Geometry: final body of the model. Coordinates: model frame, mm. Face numbers are marked on the shaded views. Give positions to 0.01 mm unless a question says otherwise; leave off trailing zeros. Loops run counter-clockwise (first coordinate to the right, second up) from the corner with the lowest first, then second, coordinate; pieces in that order, holes last.
from build123d import *

# Parameters (mm, degrees)
F0_W         = 28
F0_H         = 88.9
F0_R         = 11.5
F1_DEPTH     = 11
F2_T1_DEPTH  = 78.74
F2_T3_DEPTH  = 17.84
F2_T5_DEPTH  = 0.84
F2_S9_W      = 5.08
F2_S9_H      = 5.08
F2_T10_DEPTH = 5.08
F2_S15_W     = 5.08
F2_S15_H     = 5.08
F2_T16_DEPTH = 5.08
F2_S21_W     = 5.08
F2_S21_H     = 5.08
F2_T22_DEPTH = 5.08
F2_S27_W     = 5.08
F2_S27_H     = 5.08
F2_T28_DEPTH = 5.08
F2_S33_W     = 5.08
F2_S33_H     = 5.08
F2_T34_DEPTH = 5.08
F2_S39_W     = 5.08
F2_S39_H     = 5.08
F2_T40_DEPTH = 5.08
F2_S45_W     = 5.08
F2_S45_H     = 5.08
F2_T46_DEPTH = 5.08
F2_S51_W     = 5.08
F2_S51_H     = 5.08
F2_T52_DEPTH = 5.08


# Not quite as in the source:
# - a fillet or chamfer that OpenCascade refuses, or shapes differently, is made with other operations: its cross-section is extruded or revolved along the edge and cut away or added


with BuildPart() as f1:
    # F0 (on Top) → F1 (new body)
    with BuildSketch(Plane.XY):
        with Locations((-14, 0)):
            Rectangle(F0_W, F0_H)
        with Locations((-13.97, -26.67)):
            Circle(F0_R, mode=Mode.SUBTRACT)
        with Locations((-13.97, 0)):
            Circle(F0_R, mode=Mode.SUBTRACT)
        with Locations((-13.97, 26.67)):
            Circle(F0_R, mode=Mode.SUBTRACT)
    extrude(amount=F1_DEPTH)

    # F2: fillet of radius 5.08 on 12 edges, made by hand

    # F2_s2 → F2_t1 (cut)
    with BuildSketch(Plane.XZ.offset(-39.37)):
        with BuildLine():
            ThreePointArc((0, 5.92), (-1.4878975516, 9.5121024484), (-5.08, 11))
            Line((-5.08, 11), (0, 11))
            Line((0, 11), (0, 5.92))
        make_face()
        with BuildLine():
            ThreePointArc((0, 5.08), (-1.4878975516, 1.4878975516), (-5.08, 0))
            Line((-5.08, 0), (0, 0))
            Line((0, 0), (0, 5.08))
        make_face()
        with BuildLine():
            ThreePointArc((-28, 5.92), (-26.5121024484, 9.5121024484), (-22.92, 11))
            Line((-22.92, 11), (-28, 11))
            Line((-28, 11), (-28, 5.92))
        make_face()
        with BuildLine():
            ThreePointArc((-28, 5.08), (-26.5121024484, 1.4878975516), (-22.92, 0))
            Line((-22.92, 0), (-28, 0))
            Line((-28, 0), (-28, 5.08))
        make_face()
    extrude(amount=F2_T1_DEPTH, mode=Mode.SUBTRACT)

    # F2_s4 → F2_t3 (cut)
    with BuildSketch(Plane.YZ.offset(-22.92)):
        with BuildLine():
            ThreePointArc((-44.45, 5.92), (-42.9621024484, 9.5121024484), (-39.37, 11))
            Line((-39.37, 11), (-44.45, 11))
            Line((-44.45, 11), (-44.45, 5.92))
        make_face()
        with BuildLine():
            ThreePointArc((-44.45, 5.08), (-42.9621024484, 1.4878975516), (-39.37, 0))
            Line((-39.37, 0), (-44.45, 0))
            Line((-44.45, 0), (-44.45, 5.08))
        make_face()
        with BuildLine():
            ThreePointArc((44.45, 5.92), (42.9621024484, 9.5121024484), (39.37, 11))
            Line((39.37, 11), (44.45, 11))
            Line((44.45, 11), (44.45, 5.92))
        make_face()
        with BuildLine():
            ThreePointArc((44.45, 5.08), (42.9621024484, 1.4878975516), (39.37, 0))
            Line((39.37, 0), (44.45, 0))
            Line((44.45, 0), (44.45, 5.08))
        make_face()
    extrude(amount=F2_T3_DEPTH, mode=Mode.SUBTRACT)

    # F2_s6 → F2_t5 (cut)
    with BuildSketch(Plane.XY.offset(5.08)):
        with BuildLine():
            ThreePointArc((0, -39.37), (-1.4878975516, -42.9621024484), (-5.08, -44.45))
            Line((-5.08, -44.45), (0, -44.45))
            Line((0, -44.45), (0, -39.37))
        make_face()
        with BuildLine():
            ThreePointArc((-28, -39.37), (-26.5121024484, -42.9621024484), (-22.92, -44.45))
            Line((-22.92, -44.45), (-28, -44.45))
            Line((-28, -44.45), (-28, -39.37))
        make_face()
        with BuildLine():
            ThreePointArc((-22.92, 44.45), (-26.5121024484, 42.9621024484), (-28, 39.37))
            Line((-28, 39.37), (-28, 44.45))
            Line((-28, 44.45), (-22.92, 44.45))
        make_face()
        with BuildLine():
            ThreePointArc((0, 39.37), (-1.4878975516, 42.9621024484), (-5.08, 44.45))
            Line((-5.08, 44.45), (0, 44.45))
            Line((0, 44.45), (0, 39.37))
        make_face()
    extrude(amount=F2_T5_DEPTH, mode=Mode.SUBTRACT)


with BuildPart() as f2_tool8:
    # F2_s9 → F2_t10 (new body)
    with BuildSketch(Plane.YZ.offset(-5.08)):
        with Locations((-41.91, 8.46)):
            Rectangle(F2_S9_W, F2_S9_H)
    extrude(amount=F2_T10_DEPTH)

    # F2_s11 → F2_t12 (revolve, cut)
    with BuildSketch(Plane(origin=(-5.08, -39.37, 5.92), x_dir=(0, 0.7071067812, -0.7071067812), z_dir=(0, -0.7071067812, -0.7071067812))):
        with BuildLine():
            ThreePointArc((0, -5.08), (5.08, 0), (0, 5.08))
            Line((0, 5.08), (0, -5.08))
        make_face()
    revolve(axis=Axis((-5.08, -39.37, 5.92), (1, 0, 0)), mode=Mode.SUBTRACT)


with BuildPart() as f1_1:
    add(f1.part)

    # F2_t7: cut F2_tool8
    add(f2_tool8.part, mode=Mode.SUBTRACT)


with BuildPart() as f2_tool14:
    # F2_s15 → F2_t16 (new body)
    with BuildSketch(Plane.YZ.offset(-5.08)):
        with Locations((41.91, 8.46)):
            Rectangle(F2_S15_W, F2_S15_H)
    extrude(amount=F2_T16_DEPTH)

    # F2_s17 → F2_t18 (revolve, cut)
    with BuildSketch(Plane(origin=(-5.08, 39.37, 5.92), x_dir=(0, -0.7071067812, -0.7071067812), z_dir=(0, -0.7071067812, 0.7071067812))):
        with BuildLine():
            ThreePointArc((0, -5.08), (5.08, 0), (0, 5.08))
            Line((0, 5.08), (0, -5.08))
        make_face()
    revolve(axis=Axis((-5.08, 39.37, 5.92), (1, 0, 0)), mode=Mode.SUBTRACT)


with BuildPart() as f1_2:
    add(f1_1.part)

    # F2_t13: cut F2_tool14
    add(f2_tool14.part, mode=Mode.SUBTRACT)


with BuildPart() as f2_tool20:
    # F2_s21 → F2_t22 (new body)
    with BuildSketch(Plane.XY.offset(5.92)):
        with Locations((-25.46, -41.91)):
            Rectangle(F2_S21_W, F2_S21_H)
    extrude(amount=F2_T22_DEPTH)

    # F2_s23 → F2_t24 (revolve, cut)
    with BuildSketch(Plane(origin=(-22.92, -39.37, 5.92), x_dir=(0.7071067812, 0.7071067812, 0), z_dir=(0.7071067812, -0.7071067812, 0))):
        with BuildLine():
            ThreePointArc((0, -5.08), (5.08, 0), (0, 5.08))
            Line((0, 5.08), (0, -5.08))
        make_face()
    revolve(axis=Axis((-22.92, -39.37, 5.92), (0, 0, 1)), mode=Mode.SUBTRACT)


with BuildPart() as f1_3:
    add(f1_2.part)

    # F2_t19: cut F2_tool20
    add(f2_tool20.part, mode=Mode.SUBTRACT)


with BuildPart() as f2_tool26:
    # F2_s27 → F2_t28 (new body)
    with BuildSketch(Plane.YZ.offset(-22.92)):
        with Locations((-41.91, 2.54)):
            Rectangle(F2_S27_W, F2_S27_H)
    extrude(amount=-F2_T28_DEPTH)

    # F2_s29 → F2_t30 (revolve, cut)
    with BuildSketch(Plane(origin=(-22.92, -39.37, 5.08), x_dir=(0, 0.7071067812, 0.7071067812), z_dir=(0, -0.7071067812, 0.7071067812))):
        with BuildLine():
            ThreePointArc((0, -5.08), (5.08, 0), (0, 5.08))
            Line((0, 5.08), (0, -5.08))
        make_face()
    revolve(axis=Axis((-22.92, -39.37, 5.08), (-1, 0, 0)), mode=Mode.SUBTRACT)


with BuildPart() as f1_4:
    add(f1_3.part)

    # F2_t25: cut F2_tool26
    add(f2_tool26.part, mode=Mode.SUBTRACT)


with BuildPart() as f2_tool32:
    # F2_s33 → F2_t34 (new body)
    with BuildSketch(Plane.YZ.offset(-5.08)):
        with Locations((-41.91, 2.54)):
            Rectangle(F2_S33_W, F2_S33_H)
    extrude(amount=F2_T34_DEPTH)

    # F2_s35 → F2_t36 (revolve, cut)
    with BuildSketch(Plane(origin=(-5.08, -39.37, 5.08), x_dir=(0, 0.7071067812, 0.7071067812), z_dir=(0, 0.7071067812, -0.7071067812))):
        with BuildLine():
            ThreePointArc((0, -5.08), (5.08, 0), (0, 5.08))
            Line((0, 5.08), (0, -5.08))
        make_face()
    revolve(axis=Axis((-5.08, -39.37, 5.08), (1, 0, 0)), mode=Mode.SUBTRACT)


with BuildPart() as f1_5:
    add(f1_4.part)

    # F2_t31: cut F2_tool32
    add(f2_tool32.part, mode=Mode.SUBTRACT)


with BuildPart() as f2_tool38:
    # F2_s39 → F2_t40 (new body)
    with BuildSketch(Plane.YZ.offset(-5.08)):
        with Locations((41.91, 2.54)):
            Rectangle(F2_S39_W, F2_S39_H)
    extrude(amount=F2_T40_DEPTH)

    # F2_s41 → F2_t42 (revolve, cut)
    with BuildSketch(Plane(origin=(-5.08, 39.37, 5.08), x_dir=(0, -0.7071067812, 0.7071067812), z_dir=(0, 0.7071067812, 0.7071067812))):
        with BuildLine():
            ThreePointArc((0, -5.08), (5.08, 0), (0, 5.08))
            Line((0, 5.08), (0, -5.08))
        make_face()
    revolve(axis=Axis((-5.08, 39.37, 5.08), (1, 0, 0)), mode=Mode.SUBTRACT)


with BuildPart() as f1_6:
    add(f1_5.part)

    # F2_t37: cut F2_tool38
    add(f2_tool38.part, mode=Mode.SUBTRACT)


with BuildPart() as f2_tool44:
    # F2_s45 → F2_t46 (new body)
    with BuildSketch(Plane.XY.offset(5.92)):
        with Locations((-25.46, 41.91)):
            Rectangle(F2_S45_W, F2_S45_H)
    extrude(amount=F2_T46_DEPTH)

    # F2_s47 → F2_t48 (revolve, cut)
    with BuildSketch(Plane(origin=(-22.92, 39.37, 5.92), x_dir=(0.7071067812, -0.7071067812, 0), z_dir=(-0.7071067812, -0.7071067812, 0))):
        with BuildLine():
            ThreePointArc((0, -5.08), (5.08, 0), (0, 5.08))
            Line((0, 5.08), (0, -5.08))
        make_face()
    revolve(axis=Axis((-22.92, 39.37, 5.92), (0, 0, 1)), mode=Mode.SUBTRACT)


with BuildPart() as f1_7:
    add(f1_6.part)

    # F2_t43: cut F2_tool44
    add(f2_tool44.part, mode=Mode.SUBTRACT)


with BuildPart() as f2_tool50:
    # F2_s51 → F2_t52 (new body)
    with BuildSketch(Plane.XZ.offset(-39.37)):
        with Locations((-25.46, 2.54)):
            Rectangle(F2_S51_W, F2_S51_H)
    extrude(amount=-F2_T52_DEPTH)

    # F2_s53 → F2_t54 (revolve, cut)
    with BuildSketch(Plane(origin=(-22.92, 39.37, 5.08), x_dir=(0.7071067812, 0, 0.7071067812), z_dir=(-0.7071067812, 0, 0.7071067812))):
        with BuildLine():
            ThreePointArc((0, -5.08), (5.08, 0), (0, 5.08))
            Line((0, 5.08), (0, -5.08))
        make_face()
    revolve(axis=Axis((-22.92, 39.37, 5.08), (0, 1, 0)), mode=Mode.SUBTRACT)


with BuildPart() as f1_8:
    add(f1_7.part)

    # F2_t49: cut F2_tool50
    add(f2_tool50.part, mode=Mode.SUBTRACT)


solid = f1_8.part
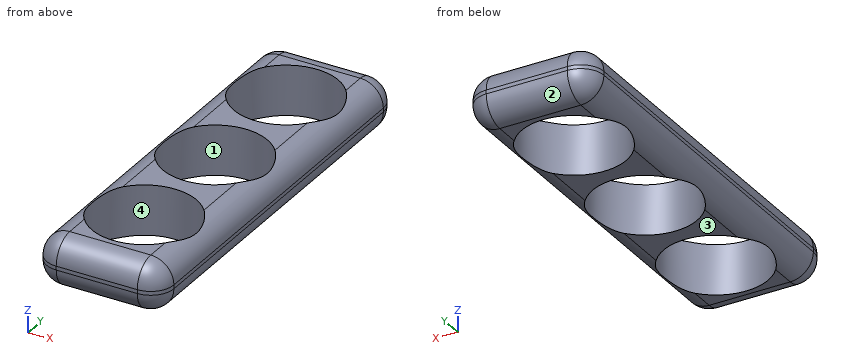
Item 1: Ray query, probe 1 along Y at (x, z) = (-13.97, 6.25); probe 2 along Y at (x, z) = (-8, 6.25); probe 3 along X at (y, z) = (28.5, 2.5). Return the intervals inside material, ascending.
Values follow:
probe 1: y = -44.44 to -38.17, -15.17 to -11.5, 11.5 to 15.17, 38.17 to 44.44
probe 2: y = -44.44 to -36.5, -16.84 to -9.83, 9.83 to 16.84, 36.5 to 44.44
probe 3: x = -27.3 to -25.32, -2.62 to -0.7
Item 2: Section query B-B on y = 0. Return loops of the section in (x, z), plus the area to 3 significant figures.
Values follow:
outline: (-28, 5.08) arc R5.08 ccw to (-25.47, 0.69) - (-25.47, 10.31) arc R5.08 ccw to (-28, 5.92) - close; (-2.47, 0.72) arc R5.08 ccw to (0, 5.08) - (0, 5.92) arc R5.08 ccw to (-2.47, 10.28) - close
area: 35.2 mm2
Item 3: Draft query along Y for the marked faces 1, 2, 3 and 4. Return one class per face: +Y half, -Y half, draft (parallel to the pull), parting line (faces both ways), or undercut.
Values follow:
face 1: undercut
face 2: +Y half
face 3: draft
face 4: undercut
Item 4: Pin query (flat end, axial travel): pin 1 (1.5 mm diameter, centred on y = -22.5, z = 7.5, fed in from -X); pin 2 (3 mm diameter, centred on y = 14, z = 2, fed in from -X); pin 3 (1 mm diameter, centred on x = -3.5, y = -22.5, fed in from +Z). Return the tip coordinate at first contact, or that it passes through.
Values follow:
pin 1: stops at x = -27.93
pin 2: stops at x = -27.75
pin 3: stops at z = 10.73
Item 5: Section query A-A on x = -13.97. Return loops of the section in (y, z).
Values follow:
outline: (-44.45, 5.08) arc R5.08 ccw to (-39.37, 0) - (-38.17, 0) - (-38.17, 11) - (-39.37, 11) arc R5.08 ccw to (-44.45, 5.92) - close; (-15.17, 0) - (-11.5, 0) - (-11.5, 11) - (-15.17, 11) - close; (11.5, 0) - (15.17, 0) - (15.17, 11) - (11.5, 11) - close; (38.17, 0) - (39.37, 0) arc R5.08 ccw to (44.45, 5.08) - (44.45, 5.92) arc R5.08 ccw to (39.37, 11) - (38.17, 11) - close
Item 6: Section query D-D on y = 13.5. Return loops of the section in (x, z).
Values follow:
outline: (-28, 5.08) arc R5.08 ccw to (-22.92, 0) - (-5.08, 0) arc R5.08 ccw to (0, 5.08) - (0, 5.92) arc R5.08 ccw to (-5.08, 11) - (-22.92, 11) arc R5.08 ccw to (-28, 5.92) - close
Item 7: Section query C-C on z = 2.25. Return loops of the section in (x, y).
Values follow:
outline: (-27.14, -39.37) arc R4.22 ccw to (-22.92, -43.59) - (-5.08, -43.59) arc R4.22 ccw to (-0.86, -39.37) - (-0.86, 39.37) arc R4.22 ccw to (-5.08, 43.59) - (-22.92, 43.59) arc R4.22 ccw to (-27.14, 39.37) - close; hole circle Ø23 at (-13.97, -26.67); hole circle Ø23 at (-13.97, 0); hole circle Ø23 at (-13.97, 26.67)
